from build123d import *

# Parameters (mm, degrees)
SKETCH1_W           = 100
SKETCH1_H           = 30
BOSS_EXTRUDE1_DEPTH = 20
CUT_EXTRUDE1_DEPTH  = 62.64414003
FILLET1_R           = 5
SKETCH3_W           = 100
SKETCH3_H           = 30
BOSS_EXTRUDE2_DEPTH = 5
SKETCH4_R           = 7.675
CUT_EXTRUDE2_DEPTH  = 5
CHAMFER1_SIZE       = 1


with BuildPart() as part:
    # Sketch1 → Boss-Extrude1 (new body)
    with BuildSketch(Plane(origin=(0, 0, 0), x_dir=(1, 0, 0), z_dir=(0, 1, 0))):
        Rectangle(SKETCH1_W, SKETCH1_H)
    extrude(amount=BOSS_EXTRUDE1_DEPTH)

    # Sketch2 → Cut-Extrude1 (cut, through all)
    with BuildSketch(Plane.XY.offset(15)):
        with BuildLine():
            Line((-50, 20), (50, 20))
            ThreePointArc((50, 20), (0, 12), (-50, 20))
        make_face()
    extrude(amount=-CUT_EXTRUDE1_DEPTH, mode=Mode.SUBTRACT)

    # Fillet1
    fillet1_edges = [part.edges().sort_by_distance(p)[0] for p in [
        (-50, 20, 0),
        (50, 20, 0),
    ]]
    fillet(fillet1_edges, radius=FILLET1_R)

    # Sketch3 → Boss-Extrude2 (add)
    with BuildSketch(Plane.XZ):
        Rectangle(SKETCH3_W, SKETCH3_H)
    extrude(amount=BOSS_EXTRUDE2_DEPTH)

    # Sketch4 → Cut-Extrude2 (cut)
    with BuildSketch(Plane.XZ.offset(5)):
        with Locations(Location((0, 0, 0), (0, 0, 270))):
            Circle(SKETCH4_R)
    extrude(amount=-CUT_EXTRUDE2_DEPTH, mode=Mode.SUBTRACT)

    # Chamfer1
    chamfer1_edges = [part.edges().sort_by_distance(p)[0] for p in [
        (0, -5, 7.675),
    ]]
    chamfer(chamfer1_edges, length=CHAMFER1_SIZE)


solid = part.part
Build history of the part. All positions in model axes, mm. A direction names the side the tool comes from. Round coordinates to 2 decimals unless told otherwise and drop trailing zeros. Write each loop counter-clockwise with the first axis right and the second up, starting at its lowest first coordinate (ties: lowest second). Pieces come first, ordered by that corner, then holes. Notation, with made-up numbers: M -17.75,50.25 L 41.25,50.25 A20 ccw 41.25,75.25 Z; hole C -10,33.5 d10. An arc over 180 degrees is marked long. Answer in a Markdown table with one row per item.
1. Saw through at D-D (x = -32). List the corners of the cut face in (y, z).
Geometry check:
| item | result |
|---|---|
| outline | M -5,-15 L 15.23,-15 L 15.23,15 L -5,15 Z |
2. Saw through at B-B (z = 0). List the corners of the cut face in (x, y) (3 decimals).
Geometry check:
| item | result |
|---|---|
| outline | M -50,-5 L -8.675,-5 L -7.675,-4 L -7.675,0 L 7.675,0 L 7.675,-4 L 8.675,-5 L 50,-5 L 50,13.245 A5 ccw 43.638,18.056 A160.25 cw -43.638,18.056 A5 ccw -50,13.245 Z |
3. Mould opens along X. For faces 3 (the face through (-1, 4, 15)), 4 (the face through (50, 4, 0)), 5 (the face through (0, 0, 0)) say: +X half, -X half, draft (parallel to the pull), parting line (faces both ways), or undercut.
Geometry check:
| item | result |
|---|---|
| face 3 | draft |
| face 4 | +X half |
| face 5 | undercut |
4. Which spindle directions (+Z, -Z, +X, -X, +Y, -Y) get a long thin tool onto all of the face, cutting with end or side? Do faces 1 (the face through (-4.67, -2.03, 6.09)), 2 (the face through (-1, 4, -15)). Say none if no direction does.
Geometry check:
| item | result |
|---|---|
| face 1 | -Y |
| face 2 | -Z, +X, -X, +Y, -Y |
5. Probe L1, parallel to X at y = -2.5, z = 0 (3 decimals); L2, parallel to Y at x = -26, z = 8.5; L3, parallel to Y at x = 43, z = 4.5. List the from-to ranges inside material, lowest first. Write a range as [from, to].
Geometry check:
| item | result |
|---|---|
| L1 | [-50, -7.675], [7.675, 50] |
| L2 | [-5, 14.12] |
| L3 | [-5, 17.88] |
6. Flat gauge pins, fed straight in: P1, Ø8, axis at x = -4, y = 15, coming from the -Z side; P2, Ø2, axis at x = -25, z = 0, coming from the +Y side; P3, Ø7.5, axis at x = -2.5, z = 1.5, coming from the -Y side. Where does each tip first touch, or does it go through?
Geometry check:
| item | result |
|---|---|
| P1 | z = -15 |
| P2 | y = 14.12 |
| P3 | y = 0 |
7. Saw through at C-C (y = 15.25). List the corners of the cut face in (x, z).
Geometry check:
| item | result |
|---|---|
| outline | M -49.58,-15 L -32.11,-15 L -32.11,15 L -49.58,15 Z; M 32.11,-15 L 49.58,-15 L 49.58,15 L 32.11,15 Z |
8. Saw through at A-A (x = 0). List the corners of the cut face in (y, z) (3 decimals).
Geometry check:
| item | result |
|---|---|
| outline | M -5,-15 L 12,-15 L 12,15 L -5,15 L -5,8.675 L -4,7.675 L 0,7.675 L 0,-7.675 L -4,-7.675 L -5,-8.675 Z |
